from build123d import *

# Parameters (mm, degrees)
SKETCH5_R          = 3
CUT_EXTRUDE2_DEPTH = 500
CIRPATTERN2_COUNT  = 8


with BuildPart() as part:
    # Sketch4 → Revolve1 (revolve)
    with BuildSketch(Plane.XY, mode=Mode.PRIVATE) as revolve1_sk:
        Polygon((19, 17), (19, -17), (31, -17), (31, -20), (16, -20), (16, 20), (31, 20), (31, 17), align=None)
    revolve(revolve1_sk.sketch.rotate(Axis((0, 0, 0), (0, 1, 0)), 90), axis=Axis((0, 0, 0), (0, 1, 0)))

    # Sketch5 → Cut-Extrude2 (cut, symmetric)
    with BuildSketch(Plane(origin=(0, -17, 0), x_dir=(1, 0, 0), z_dir=(0, 1, 0))):
        with Locations(Location((25, 0, 0), (0, 0, 90))):
            Circle(SKETCH5_R)
    cut_extrude2 = extrude(amount=CUT_EXTRUDE2_DEPTH, both=True, mode=Mode.SUBTRACT)

    # CirPattern2: Cut-Extrude2 ×8 about axis
    cirpattern2_axis = Axis((0, 0, 0), (0, 1, 0))
    for i in range(1, CIRPATTERN2_COUNT):
        add(cut_extrude2.rotate(cirpattern2_axis, i * 360 / CIRPATTERN2_COUNT), mode=Mode.SUBTRACT)


solid = part.part
The listing builds one solid part. Answer for the finished solid, in the listing's coordinates (mm). A direction names the side the tool comes from. Coordinates: 2 decimals unless noted, no trailing zeros. Write each loop counter-clockwise with the first axis right and the second up, starting at its lowest first coordinate (ties: lowest second). Pieces come first, ordered by that corner, then holes. Notation, with made-up numbers: (15.25, 30.5) - (65.25, 30.5) arc R18 cw to (65.25, 43.5) - close; hole circle Ø4 at (38.25, 85). An arc over 180 degrees is marked (long way). Answer as CSV lines item,"result".
1. Given P1, Ø12, axis at y = 4, z = 6, coming from the +X side; P2, Ø3, axis at y = -2, z = 18, coming from the +X side; P3, Ø1, axis at y = 3, z = -14, coming from the +X side, each flat-ended and moving along its own axis, determine where each tip first touches the part or whether it passes through.
Computed values:
P1,"stops at x = 19"
P2,"stops at x = 9.42"
P3,"stops at x = 13.37"
2. Determine the mould class of faces 3 (the flat face through (13, -20, -13)), 4 (the cylindrical face through (24.1, 18.52, -2.86)), 5 (the cylindrical face through (-30.736, 18.479, 4.036)) for opening direction Z: +Z half, -Z half, draft (parallel to the pull), parting line (faces both ways), or undercut.
Computed values:
face 3,"draft"
face 4,"undercut"
face 5,"parting line"
3. A tool of negligible diameter and unlimited length cuts with its end or side. For faces 1 (the flat face through (-14.2, -17, 13.3)), 2 (the cylindrical face through (24.1, -18.48, -2.86)), from which of +Z, -Z, +X, -X, +Y, -Y can it reach the whole face along a straight path? Write none if from no direction.
Computed values:
face 1,"none"
face 2,"+Y, -Y"
4. Find section C-C (x = 24). Give the vertices of the cut face in (y, z).
Computed values:
outline,"(-20, -19.62) - (-17, -19.62) - (-17, -2.83) - (-20, -2.83) - close; (-20, 2.83) - (-17, 2.83) - (-17, 19.62) - (-20, 19.62) - close; (17, -19.62) - (20, -19.62) - (20, -2.83) - (17, -2.83) - close; (17, 2.83) - (20, 2.83) - (20, 19.62) - (17, 19.62) - close"
5. Find section D-D (z = 25). Give the vertices of the cut face in (x, y).
Computed values:
outline,"(-18.33, -20) - (-3, -20) - (-3, -17) - (-18.33, -17) - close; (-18.33, 17) - (-3, 17) - (-3, 20) - (-18.33, 20) - close; (3, -20) - (18.33, -20) - (18.33, -17) - (3, -17) - close; (3, 17) - (18.33, 17) - (18.33, 20) - (3, 20) - close"
6. Find section A-A (x = 0). Give the number of separate pieces and of enclosed holes in the cut face, plus the area to 3 significant figures.
Computed values:
separate pieces,"6"
enclosed holes,"0"
area,"312 mm²"
7. Straight lines are drawn through the part: line 1 (Y direction, x = -6, z = -21); line 2 (X direction, y = 18, z = 0); line 3 (X direction, y = 1, z = 0). For each, find the intervals that lie inside material, in ascending order. Write a range as [from, to].
Computed values:
line 1,"y = [-20, -17], [17, 20]"
line 2,"x = [-31, -28], [-22, -16], [16, 22], [28, 31]"
line 3,"x = [-19, -16], [16, 19]"
